Check sheet for the modelled part. Datum: model origin and axes. Units: mm. A direction names the side the tool comes from. Round coordinates to 2 decimals unless told otherwise and drop trailing zeros. Order: outer loops, then holes, each group sorted by start corner. A loop starts at its lowest first (then second) coordinate and runs counter-clockwise, first axis right, second up.
(1) Mould release check, pull along Y, two halves, no side actions. Record for faces 1 (the cylindrical face through (-24.6, 22.8, 4.6)), 2 (the cylindrical face through (24.43, 29.4, 5.92)), 3 (the flat face through (-25, -23, 9)): released by +Y, released by -Y, zero draft, split by the parting line, or undercut.
(2) Thickness scan on probe 1 along X at (y, z) = (0.5, 3.5) (3 decimals); probe 2 along Y at (x, z) = (0, 0.65); probe 3 along X at (y, z) = (13, 10). Record the ranges inside material, lowest first.
(3) Depth check by flat-ended pin: pin 1 (5 mm diameter, centred on x = -3, y = 9, fed in from +Z); pin 2 (1.5 mm diameter, centred on x = 16.5, z = 10, fed in from -Y); pin 3 (0.9 mm diameter, centred on x = -25.5, y = -23, fed in from +Z). Enter the tip coordinate at first touch or a pass-through.
(4) Sectioned sample at C-C, the plane x = 11. Enter the section's corners in (y, z), and give its area (3 significant figures).
(5) Sectioned sample at A-A, the plane y = 0. Enter the section's corners in (x, z), and give its area (3 significant figures).
(6) Sectioned sample at D-D, the plane y = 14. Enter the section's corners in (x, z), and give its area (3 significant figures).
(7) Tool access check on faces 4 (the flat face through (-21.5, -24, 11)), 5 (the flat face through (-32, -21, 7)), 6 (the flat face through (20, 29, 6)), 7 (the flat face through (-32, 22, 2)). Record the directions out of +Z, -Z, +X, -X, +Y, -Y that give a thin tool (end or side, any length) a straight path to the whole face; none if there is none.
(8) Sectioned sample at B-B, the plane x = 3.5. Enter the section's corners in (y, z) (3 decimals), and give its area (3 significant figures).
```python
from build123d import *

# Parameters (mm, degrees)
SKETCH_R        = 6
PAD_DEPTH       = 12
POCKET_DEPTH    = 10.5
FILLET_R        = 9
POCKET001_DEPTH = 12.001
SKETCH003_W     = 6
SKETCH003_H     = 40
POCKET002_DEPTH = 10.5
POCKET003_DEPTH = 10
SKETCH005_R     = 4
SKETCH005_R_2   = 3
SKETCH005_W     = 6
SKETCH005_H     = 3
SKETCH005_H_2   = 3.266556
POCKET004_DEPTH = 3
SKETCH006_W     = 13
SKETCH006_H     = 9
POCKET005_DEPTH = 5
POCKET006_DEPTH = 10.5
SKETCH008_W     = 15
SKETCH008_H     = 3
POCKET007_DEPTH = 1.5
SKETCH009_W     = 15
SKETCH009_H     = 3
PAD001_DEPTH    = 1.5
POCKET008_DEPTH = 3
FILLET001_R     = 0.25
SKETCH011_R     = 2
POCKET009_DEPTH = 9.001
CHAMFER_SIZE    = 1


with BuildPart() as part:
    # Sketch → Pad (new body)
    with BuildSketch(Plane.XY):
        with BuildLine():
            ThreePointArc((-33, 30), (-34.414214, 29.414214), (-35, 28))
            Line((-35, -23), (-35, 28))
            ThreePointArc((-35, -23), (-34.414214, -24.414214), (-33, -25))
            Line((23, -25), (-33, -25))
            ThreePointArc((23, -25), (24.414214, -24.414214), (25, -23))
            Line((25, 28), (25, -23))
            ThreePointArc((25, 28), (24.414214, 29.414214), (23, 30))
            Line((-33, 30), (23, 30))
        make_face()
        Circle(SKETCH_R, mode=Mode.SUBTRACT)
    extrude(amount=PAD_DEPTH)

    # Sketch001 (on Face11 of Pad) → Pocket (cut)
    with BuildSketch(Plane.XY.offset(12)):
        with BuildLine():
            ThreePointArc((0, -23), (7.785306, 21.642297), (-14.651471, -17.729479))
            ThreePointArc((-15.925512, -19.271172), (-14.517644, -19.137346), (-14.651471, -17.729479))
            ThreePointArc((-4.974937, 24.5), (-24.252548, 6.067448), (-15.925512, -19.271172))
            Line((-4.974937, 24.5), (25, 24.5))
            Line((25, 24.5), (25, 27))
            Line((25, 27), (-5.220153, 27))
            ThreePointArc((-5.220153, 27), (-26.980945, 5.317761), (-15.074813, -23))
            Line((-15.074813, -23), (0, -23))
        make_face()
    extrude(amount=-POCKET_DEPTH, mode=Mode.SUBTRACT)

    # Fillet
    fillet_edges = [part.edges().sort_by_distance(p)[0] for p in [
        (-15.074813, -23, 6.75),
    ]]
    fillet(fillet_edges, radius=FILLET_R)

    # Sketch002 (on Face1 of Fillet) → Pocket001 (cut, through all)
    with BuildSketch(Plane.XY.offset(12)):
        with BuildLine():
            ThreePointArc((24, -17.5), (22.75, -18.75), (24, -20))
            Line((24, -20), (25, -20))
            Line((25, -17.5), (25, -20))
            Line((24, -17.5), (25, -17.5))
        make_face()
    extrude(amount=-POCKET001_DEPTH, mode=Mode.SUBTRACT)

    # Sketch003 (on Face1 of Pocket001) → Pocket002 (cut)
    with BuildSketch(Plane.XY.offset(12)):
        with Locations((-32, -1)):
            Rectangle(SKETCH003_W, SKETCH003_H)
    extrude(amount=-POCKET002_DEPTH, mode=Mode.SUBTRACT)

    # Sketch004 (on Face1 of Pocket002) → Pocket003 (cut)
    with BuildSketch(Plane.XY.offset(12)):
        Polygon((-33, 22), (-33, 19), (-30, 19), (-30, 22), (-29.5, 25), (-33.5, 25), align=None)
    extrude(amount=-POCKET003_DEPTH, mode=Mode.SUBTRACT)

    # Sketch005 (on Face1 of Pocket003) → Pocket004 (cut)
    with BuildSketch(Plane.XY.offset(12)):
        with Locations((-23, 24)):
            Circle(SKETCH005_R)
        with Locations((20.5, 20)):
            Circle(SKETCH005_R_2)
        with Locations((-24.5, -23.5)):
            Rectangle(SKETCH005_W, SKETCH005_H)
        with Locations((17.5, -23.366722)):
            Rectangle(SKETCH005_W, SKETCH005_H_2)
    extrude(amount=-POCKET004_DEPTH, mode=Mode.SUBTRACT)

    # Sketch006 (on Face32 of Pocket004) → Pocket005 (cut)
    with BuildSketch(Plane(origin=(0, 30, 0), x_dir=(-1, 0, 0), z_dir=(0, 1, 0))):
        with Locations((-13.5, 6)):
            Rectangle(SKETCH006_W, SKETCH006_H)
    extrude(amount=-POCKET005_DEPTH, mode=Mode.SUBTRACT)

    # Sketch007 (on Face1 of Pocket005) → Pocket006 (cut)
    with BuildSketch(Plane.XY.offset(12)):
        Polygon((7, 27.75), (-8, 30), (-4.666667, 30), (7, 28.25), align=None)
    extrude(amount=-POCKET006_DEPTH, mode=Mode.SUBTRACT)

    # Sketch008 (on Face1 of Pocket006) → Pocket007 (cut)
    with BuildSketch(Plane.XY.offset(12)):
        with Locations((-0.5, 28.5)):
            Rectangle(SKETCH008_W, SKETCH008_H)
    extrude(amount=-POCKET007_DEPTH, mode=Mode.SUBTRACT)

    # Sketch009 (on Face54 of Pocket007) → Pad001 (join)
    with BuildSketch(Plane.XY.offset(10.5)):
        with Locations((-0.5, 28.5)):
            Rectangle(SKETCH009_W, SKETCH009_H)
    extrude(amount=PAD001_DEPTH)

    # Sketch010 (on Face45 of Pad001) → Pocket008 (cut)
    with BuildSketch(Plane.XY.offset(12)):
        with BuildLine():
            Line((-24.5, 30), (-24.5, 27.708099))
            ThreePointArc((-21.5, 27.708099), (-23, 28), (-24.5, 27.708099))
            Line((-21.5, 27.708099), (-21.5, 30))
            Line((-21.5, 30), (-24.5, 30))
        make_face()
        with BuildLine():
            Line((23.098076, 18.5), (25, 18.5))
            Line((25, 18.5), (25, 21.5))
            Line((25, 21.5), (23.098076, 21.5))
            ThreePointArc((23.098076, 18.5), (23.5, 20), (23.098076, 21.5))
        make_face()
    extrude(amount=-POCKET008_DEPTH, mode=Mode.SUBTRACT)

    # Fillet001
    fillet001_edges = [part.edges().sort_by_distance(p)[0] for p in [
        (-4.666667, 30, 6),
    ]]
    fillet(fillet001_edges, radius=FILLET001_R)

    # Sketch011 (on Face24 of Fillet001) → Pocket009 (cut, through all)
    with BuildSketch(Plane.XY.offset(9)):
        with Locations((-23, 24)):
            Circle(SKETCH011_R)
        with Locations((20.5, 20)):
            Circle(SKETCH011_R)
    extrude(amount=-POCKET009_DEPTH, mode=Mode.SUBTRACT)

    # Chamfer
    chamfer_edges = [part.edges().sort_by_distance(p)[0] for p in [
        (-29, 19, 6.75),
    ]]
    chamfer(chamfer_edges, length=CHAMFER_SIZE)


solid = part.part
```
Derived:
1. face 1: undercut
1. face 2: released by +Y
1. face 3: zero draft
2. probe 1: x = -29 to -27.495, -24.995 to -22.995, 22.995 to 25
2. probe 2: y = -25 to -6, 6 to 30
2. probe 3: x = -29 to -24.23, -21.35 to -18.97, 18.97 to 25
3. pin 1: stops at z = 1.5
3. pin 2: stops at y = -21.73
3. pin 3: stops at z = 9
4. outline: (-25, 0) - (30, 0) - (30, 1.5) - (24.5, 1.5) - (24.5, 12) - (20.2, 12) - (20.2, 1.5) - (-20.2, 1.5) - (-20.2, 12) - (-25, 12) - close; (27, 10.5) - (30, 10.5) - (30, 12) - (27, 12) - close
4. area: 183 mm2
5. outline: (-35, 0) - (-6, 0) - (-6, 1.5) - (-23, 1.5) - (-23, 12) - (-25, 12) - (-25, 1.5) - (-27.5, 1.5) - (-27.5, 12) - (-29, 12) - (-29, 1.5) - (-35, 1.5) - close; (6, 0) - (25, 0) - (25, 12) - (23, 12) - (23, 1.5) - (6, 1.5) - close
5. area: 130 mm2
6. outline: (-35, 0) - (25, 0) - (25, 12) - (18.25, 12) - (18.25, 1.5) - (-18.25, 1.5) - (-18.25, 12) - (-20.71, 12) - (-20.71, 1.5) - (-23.67, 1.5) - (-23.67, 12) - (-29, 12) - (-29, 1.5) - (-35, 1.5) - close
6. area: 243 mm2
7. face 4: +Z, -Y
7. face 5: +Z, -X
7. face 6: +Y
7. face 7: +Z
8. outline: (-25, 0) - (-4.873, 0) - (-4.873, 1.5) - (-22.732, 1.5) - (-22.732, 12) - (-25, 12) - close; (4.873, 0) - (30, 0) - (30, 12) - (27, 12) - (27, 1.5) - (24.5, 1.5) - (24.5, 12) - (22.732, 12) - (22.732, 1.5) - (4.873, 1.5) - close; hole (28.275, 1.5) - (28.775, 1.5) - (28.775, 10.5) - (28.275, 10.5) - close
8. area: 137 mm2
